Autodesk Fusion 360 part; units mm, degrees
sketch "Sketch1" plane through (0, 0, 0) normal (0, 0, 1) x (1, 0, 0)
  line L0 (0, 0) -> (139.7, 0)
  line L1 (139.7, 0) -> (139.7, 25)
  line L2 (139.7, 25) -> (0, 25)
  line L3 (0, 25) -> (0, 0)
  dimension "d1" = 139.7
  dimension "d2" = 25
extrude "Extrude1" add sketch "Sketch1" along normal blind 5
sketch "Sketch2" plane through (0, 0, 0) normal (0, 0, 1) x (1, 0, 0)
  point P0 (6.35, 12.5)
  point P1 (133.35, 12.5)
hole "Hole1" at (6.35, 12.5, 0) at (133.35, 12.5, 0) direction (0, 0, 1) diameter 5.5 depth 13 tip angle 118 counterbore diameter 9.1 counterbore depth 1
sketch "Sketch5" plane through (0, 0, 0) normal (0, 0, -1) x (1, 0, 0)
  circle A0 centre (6.35, -12.5) radius 4.55
  circle A1 centre (133.35, -12.5) radius 4.55
  line L0 (0, 0) -> (0, -25)
  line L1 (0, -25) -> (139.7, -25)
  line L2 (139.7, -25) -> (139.7, 0)
  line L3 (139.7, 0) -> (0, 0)
  point P0 (69.85, -12.5)
hole "Hole4" at (69.85, 12.5, 0) direction (0, 0, 1) diameter 3.75 depth 15 tip angle 118
Source: CAD feature listing. Evaluate the final solid. Frame: model axes, mm. A direction names the side the tool comes from. Coordinates: 2 decimals unless noted, no trailing zeros. Write each loop counter-clockwise with the first axis right and the second up, starting at its lowest first coordinate (ties: lowest second). Pieces come first, ordered by that corner, then holes. Notation, with made-up numbers: (-21, 71.25) - (3, 71.25) arc R29 cw to (3, 104.25) - close; hole circle Ø8 at (17, 23.25). An arc over 180 degrees is marked (long way). Answer as a JSON object with one key per item and string values.
Q1. Section query C-C, the plane z = 3.6. Output: boundary loops of the cut face in (x, y) (3 decimals), plus the area to 3 significant figures.
Ans:
{"outline": "(0, 0) - (139.7, 0) - (139.7, 25) - (0, 25) - close; hole circle Ø5.5 at (6.35, 12.5); hole circle Ø3.75 at (69.85, 12.5); hole circle Ø5.5 at (133.35, 12.5)", "area": "3,430 mm2"}
Q2. Section query A-A, the plane y = 12.5. Output: boundary loops of the cut face in (x, z) (3 decimals).
Ans:
{"outline": "(0, 0) - (1.8, 0) - (1.8, 1) - (3.6, 1) - (3.6, 5) - (0, 5) - close; (9.1, 1) - (10.9, 1) - (10.9, 0) - (67.975, 0) - (67.975, 5) - (9.1, 5) - close; (71.725, 0) - (128.8, 0) - (128.8, 1) - (130.6, 1) - (130.6, 5) - (71.725, 5) - close; (136.1, 1) - (137.9, 1) - (137.9, 0) - (139.7, 0) - (139.7, 5) - (136.1, 5) - close"}
Q3. Section query D-D, the plane x = 69.85. Output: boundary loops of the cut face in (y, z) (3 decimals).
Ans:
{"outline": "(0, 0) - (10.625, 0) - (10.625, 5) - (0, 5) - close; (14.375, 0) - (25, 0) - (25, 5) - (14.375, 5) - close"}
Q4. Draft query along X for faces 3 (the flat face through (139.7, 12, 2)), 4 (the flat face through (69, 15, 5)), 5 (the flat face through (9.3, 12.4, 1)). Return one class per face: released by +X, released by -X, zero draft, split by the parting line, or undercut.
Ans:
{"face 3": "released by +X", "face 4": "zero draft", "face 5": "undercut"}
Q5. Material intervals for line 1 (X direction, y = 12.5, z = 0.2) (3 decimals); line 2 (X direction, y = 12.5, z = 2.6) (3 decimals); line 3 (Y direction, x = 6.35, z = 0.5), sorted ascending. Write a range as [from, to].
Ans:
{"line 1": "x = [0, 1.8], [10.9, 67.975], [71.725, 128.8], [137.9, 139.7]", "line 2": "x = [0, 3.6], [9.1, 67.975], [71.725, 130.6], [136.1, 139.7]", "line 3": "y = [0, 7.95], [17.05, 25]"}
Q6. Set-up query: faces 1 (the cylindrical face through (2.513, 14.946, 0.507)), 2 (the cylindrical face through (71.68, 12.09, 2.54)). Return all of +Z, -Z, +X, -X, +Y, -Y with unobstructed straight access to the full face (end or side cutting, diameter ignored); none if empty.
Ans:
{"face 1": "-Z", "face 2": "+Z, -Z"}
Q7. Section query B-B, the plane x = 133.35. Output: boundary loops of the cut face in (y, z), plus the area to 3 significant figures.
Ans:
{"outline": "(0, 0) - (7.95, 0) - (7.95, 1) - (9.75, 1) - (9.75, 5) - (0, 5) - close; (15.25, 1) - (17.05, 1) - (17.05, 0) - (25, 0) - (25, 5) - (15.25, 5) - close", "area": "93.9 mm2"}
